Geometry: final body of the model. Coordinates: model frame, mm. A direction names the side the tool comes from. Coordinates: 2 decimals unless noted, no trailing zeros. Loops run counter-clockwise (first coordinate to the right, second up) from the corner with the lowest first, then second, coordinate; pieces in that order, holes last. Notation, with made-up numbers: (-1.75, 80.5) - (45.25, 80.5) arc R21 ccw to (45.25, 106.5) - close; hole circle Ø6 at (84.5, 78.5). An arc over 180 degrees is marked (long way). Put each result on its own line as item: value. Start each with the question number.
1) Section D-D on z = 16. Output: boundary loops of the cut face in (x, y), and give its area (3 significant figures).
2) Draft query along Z for faces 1 (the flat face through (184, 270, -55)), 2 (the flat face through (182.45, 193.95, -66.07)), 3 (the flat face through (184.137, 53.853, -193.276)), 4 (the flat face through (182.45, 196.05, -31.29)). Return one class per face: +Z half, -Z half, draft (parallel to the pull), parting line (faces both ways), or undercut.
3) Section B-B on y = 137. Output: boundary loops of the cut face in (x, z).
4) Contact query for flat-ended pins moving along their axis: pin 1 Ø0.9 at (x, y) = (13.5, 268.5) entering from +Z; pin 2 Ø3.5 at (x, y) = (359, 268) entering from -Z; pin 3 Ø12 at (x, y) = (216.5, 88) entering from +Z; pin 4 Ø10 at (y, z) = (92, -19.5) entering from -X. Output: stop coordinate, or through.
5) Reachability of faces 5 (the flat face through (367, 179, -50)), 6 (the flat face through (367, 143, -107)) from +Z, -Z, +X, -X, +Y, -Y: full face, straight path, thin tool, end or side. Return the list, or none.
6) Section A-A on x = 117. Output: boundary loops of the cut face in (y, z).
7) Section C-C on y = 37. Output: boundary loops of the cut face in (x, z), and give its area (3 significant figures).
8) Material intervals for line 1 along X through (y, z) = (269, -106) (3 decimals); line 2 along X through (y, z) = (135, -35); line 3 along Z through (x, y) = (73, 257), sorted ascending. Write a range as from..to.
```python
from build123d import *

# Parameters (mm, degrees)
BOSS_EXTRUDE1_DEPTH = 370
SHELL1_T            = -3
SKETCH4_W           = 364
SKETCH4_H           = 96.095905324
CUT_EXTRUDE2_DEPTH  = 497.302890263
BOSS_EXTRUDE2_REACH = 497.698
SKETCH9_W           = 15
SKETCH9_H           = 10
SKETCH9_R           = 2.5
BOSS_EXTRUDE4_DEPTH = 3
BOSS_EXTRUDE5_DEPTH = 4
BOSS_EXTRUDE6_DEPTH = 4
CUT_EXTRUDE3_DEPTH  = 498.923245976


with BuildPart() as part:
    # Sketch2 → Boss-Extrude1 (new body)
    with BuildSketch(Plane(origin=(0, 0, 0), x_dir=(0, 0, -1), z_dir=(1, 0, 0))):
        Polygon((100, 0), (195.262794416, 55), (100, 270), (0, 270), (-95.262794416, 55), (0, 0), (18.222222222, 120), (81.777777778, 120), align=None)
    extrude(amount=BOSS_EXTRUDE1_DEPTH)

    # Shell1
    shell1_openings = [part.faces().sort_by_distance(p)[0] for p in [
        (185, 27.5, 47.631397208),
        (185, 27.5, -147.631397208),
        (185, 60, -90.888888889),
        (185, 120, -50),
        (185, 60, -9.111111111),
    ]]
    offset(amount=SHELL1_T, openings=shell1_openings, kind=Kind.INTERSECTION)

    # Sketch4 → Cut-Extrude2 (cut, through all)
    with BuildSketch(Plane.XZ.offset(-267)):
        with Locations((185, -50)):
            Rectangle(SKETCH4_W, SKETCH4_H)
    extrude(amount=-CUT_EXTRUDE2_DEPTH, mode=Mode.SUBTRACT)

    # Sketch5 → Boss-Extrude2 (add, up to next)
    with BuildSketch(Plane(origin=(3, 0, 0), x_dir=(0, 0, -1), z_dir=(1, 0, 0)), mode=Mode.PRIVATE) as boss_extrude2_sk1:
        Polygon((47, 270), (44, 270), (18.222222222, 120), (21.222222222, 120), align=None)
    boss_extrude2_tool1 = extrude(boss_extrude2_sk1.sketch, amount=BOSS_EXTRUDE2_REACH, mode=Mode.PRIVATE) - part.part
    # Sketch5 → Boss-Extrude2 (add, up to next)
    with BuildSketch(Plane(origin=(3, 0, 0), x_dir=(0, 0, -1), z_dir=(1, 0, 0)), mode=Mode.PRIVATE) as boss_extrude2_sk2:
        Polygon((53, 270), (56, 270), (81.777777778, 120), (78.777777778, 120), align=None)
    boss_extrude2_tool2 = extrude(boss_extrude2_sk2.sketch, amount=BOSS_EXTRUDE2_REACH, mode=Mode.PRIVATE) - part.part
    add(boss_extrude2_tool1.solids().sort_by_distance((3, 195, -32.611111))[0])
    add(boss_extrude2_tool2.solids().sort_by_distance((3, 195, -67.388889))[0])

    # Sketch9 → Boss-Extrude4 (add)
    # profile 1 of 6: a face of its own
    with BuildSketch(Plane(origin=(0, 267, 0), x_dir=(1, 0, 0), z_dir=(0, 1, 0))):
        with Locations((11.965, 105)):
            Rectangle(SKETCH9_W, SKETCH9_H)
        with Locations(Location((11.965, 106, 0), (0, 0, 270))):
            Circle(SKETCH9_R, mode=Mode.SUBTRACT)
    # profile 2 of 6: a face of its own
    with BuildSketch(Plane(origin=(0, 267, 0), x_dir=(1, 0, 0), z_dir=(0, 1, 0))):
        with Locations((185.002, 105)):
            Rectangle(SKETCH9_W, SKETCH9_H)
        with Locations(Location((185.002, 106, 0), (0, 0, 270))):
            Circle(SKETCH9_R, mode=Mode.SUBTRACT)
    # profile 3 of 6: a face of its own
    with BuildSketch(Plane(origin=(0, 267, 0), x_dir=(1, 0, 0), z_dir=(0, 1, 0))):
        with Locations((358.035, 105)):
            Rectangle(SKETCH9_W, SKETCH9_H)
        with Locations(Location((358.035, 106, 0), (0, 0, 270))):
            Circle(SKETCH9_R, mode=Mode.SUBTRACT)
    # profile 4 of 6: a face of its own
    with BuildSketch(Plane(origin=(0, 267, 0), x_dir=(1, 0, 0), z_dir=(0, 1, 0))):
        with Locations((358.035, -5)):
            Rectangle(SKETCH9_W, SKETCH9_H)
        with Locations(Location((358.035, -6, 0), (0, 0, 270))):
            Circle(SKETCH9_R, mode=Mode.SUBTRACT)
    # profile 5 of 6: a face of its own
    with BuildSketch(Plane(origin=(0, 267, 0), x_dir=(1, 0, 0), z_dir=(0, 1, 0))):
        with Locations((185.002, -5)):
            Rectangle(SKETCH9_W, SKETCH9_H)
        with Locations(Location((185.002, -6, 0), (0, 0, 270))):
            Circle(SKETCH9_R, mode=Mode.SUBTRACT)
    # profile 6 of 6: a face of its own
    with BuildSketch(Plane(origin=(0, 267, 0), x_dir=(1, 0, 0), z_dir=(0, 1, 0))):
        with Locations((11.965, -5)):
            Rectangle(SKETCH9_W, SKETCH9_H)
        with Locations(Location((11.965, -6, 0), (0, 0, 270))):
            Circle(SKETCH9_R, mode=Mode.SUBTRACT)
    extrude(amount=BOSS_EXTRUDE4_DEPTH)

    # Sketch11 → Boss-Extrude5 (add)
    with BuildSketch(Plane.ZY.offset(-367)):
        Polygon((-9.111111111, 60), (-8.883333333, 58.5), (92.396882217, 61.468119339), (91.789234305, 62.839528838), align=None)
        Polygon((94.383691773, 56.984059669), (93.719067626, 58.484059669), (-8.433126527, 55.535223468), (-8.205348749, 54.035223468), align=None)
        Polygon((-191.789234305, 62.839528838), (-90.888888889, 60), (-91.116666667, 58.5), (-192.396882217, 61.468119339), align=None)
        Polygon((-194.383691773, 56.984059669), (-193.719067625, 58.484059669), (-91.566873473, 55.535223468), (-91.794651251, 54.035223468), align=None)
    extrude(amount=BOSS_EXTRUDE5_DEPTH)

    # Sketch10 → Boss-Extrude6 (add)
    with BuildSketch(Plane(origin=(3, 0, 0), x_dir=(0, 0, -1), z_dir=(1, 0, 0))):
        Polygon((9.111111111, 60), (-91.789234305, 62.839528838), (-92.396882217, 61.468119339), (8.883333333, 58.5), align=None)
        Polygon((-93.719067626, 58.484059669), (8.433126527, 55.535223468), (8.205348749, 54.035223468), (-94.383691773, 56.984059669), align=None)
        Polygon((194.383691773, 56.984059669), (193.719067625, 58.484059669), (91.566873473, 55.535223468), (91.794651251, 54.035223468), align=None)
        Polygon((192.396882217, 61.468119339), (91.116666667, 58.5), (90.888888889, 60), (191.789234305, 62.839528838), align=None)
    extrude(amount=BOSS_EXTRUDE6_DEPTH)

    # Sketch12 → Cut-Extrude3 (cut, through all)
    with BuildSketch(Plane(origin=(370, 0, 0), x_dir=(0, 0, -1), z_dir=(1, 0, 0))):
        Polygon((11.466336894, 75.51002345), (6.523006166, 76.260677375), (5.021698316, 66.37401592), (9.965029044, 65.623361994), (10.715682969, 70.566692722), align=None)
        Polygon((89.284317031, 70.566692722), (88.533663106, 75.51002345), (93.476993834, 76.260677375), (94.978301684, 66.37401592), (90.034970956, 65.623361994), align=None)
    extrude(amount=-CUT_EXTRUDE3_DEPTH, mode=Mode.SUBTRACT)


solid = part.part
```
Answer block:
1. outline: (0, 9.24) - (3, 9.24) - (3, 54.73) - (7, 54.73) - (7, 56.24) - (3, 56.24) - (3, 59.23) - (7, 59.23) - (7, 60.71) - (3, 60.71) - (3, 226.48) - (367, 226.48) - (367, 60.71) - (363, 60.71) - (363, 59.23) - (367, 59.23) - (367, 56.24) - (363, 56.24) - (363, 54.73) - (367, 54.73) - (367, 9.24) - (370, 9.24) - (370, 233.89) - (0, 233.89) - close
1. area: 4,070 mm²
2. face 1: draft
2. face 2: undercut
2. face 3: -Z half
2. face 4: undercut
3. outline: (0, -158.93) - (370, -158.93) - (370, 58.93) - (0, 58.93) - close; hole (3, -155.65) - (367, -155.65) - (367, -78.86) - (3, -78.86) - close; hole (3, -75.86) - (367, -75.86) - (367, -24.14) - (3, -24.14) - close; hole (3, -21.14) - (367, -21.14) - (367, 55.65) - (3, 55.65) - close
4. pin 1: stops at z = 10
4. pin 2: stops at z = -110
4. pin 3: stops at z = 83.3
4. pin 4: passes through
5. face 5: -Y
5. face 6: none
6. outline: (53.49, -192.65) - (55, -195.26) - (270, -100) - (270, -98.05) - (267, -98.05) - close; (53.49, 92.65) - (267, -1.95) - (270, -1.95) - (270, 0) - (55, 95.26) - close; (120, -81.78) - (270, -56) - (270, -53) - (120, -78.78) - close; (120, -21.22) - (270, -47) - (270, -44) - (120, -18.22) - close
7. outline: (0, -164.09) - (3, -164.09) - (3, -94.38) - (0, -94.38) - close; (0, -5.62) - (3, -5.62) - (3, 64.09) - (0, 64.09) - close; (367, -164.09) - (370, -164.09) - (370, -94.38) - (367, -94.38) - close; (367, -5.62) - (370, -5.62) - (370, 64.09) - (367, 64.09) - close
7. area: 836 mm²
8. line 1: x = 4.465..9.465, 14.465..19.465, 177.502..182.502, 187.502..192.502, 350.535..355.535, 360.535..365.535
8. line 2: x = 0..3, 367..370
8. line 3: z = -105.76..-102.48, -58.23..-55.23, -44.77..-41.77, 2.48..5.76
